Geometry: see drawing. Coordinates: mm, zero at the bounding-box minimum. Coordinates: 2 decimals unless noted, no trailing zeros. Write each loop counter-clockwise with the first axis right and the second up, starting at its lowest first coordinate (ties: lowest second). Pieces come first, ordered by that corner, then holes. Notation, with made-up numbers: M -33.75,-9 L -21.75,-9 A36 cw -21.75,26 Z; hole C 85,-28.75 d1. An arc over 180 degrees is marked long. One line per item, written item: value. Start each with the question number.
Item 1: Mould query, pull axis X, two halves, no side actions, for the marked faces 1, 2, 3 and 4. Classes: released by +X, released by -X, zero draft, split by the parting line, or undercut.
Item 2: Cut plane C-C, the plane y = 3.5. Output: boundary loops of the cut face in (x, z), then the cut area to 3 significant figures.
Item 3: Pin query (flat end, axial travel): P1, Ø6, axis at x = 12.5, y = 15.5, coming from the -Z side. Return the tip coordinate at first contact, or that it passes through.
Item 4: Cut plane A-A, the plane x = 12.5. Output: boundary loops of the cut face in (y, z).
Item 5: Cut plane D-D, the plane y = 15.25. Output: boundary loops of the cut face in (x, z).
Item 6: Ray query, L1, parallel to Y at x = 12.5, z = 24.5; L2, parallel to Y at x = 20.5, z = 10.5; L3, parallel to Y at x = 21, z = 16.75. Return the intervals inside material, ascending. Write a range as from..to.
Item 7: Cut plane B-B, the plane z = 15. Output: boundary loops of the cut face in (x, y).
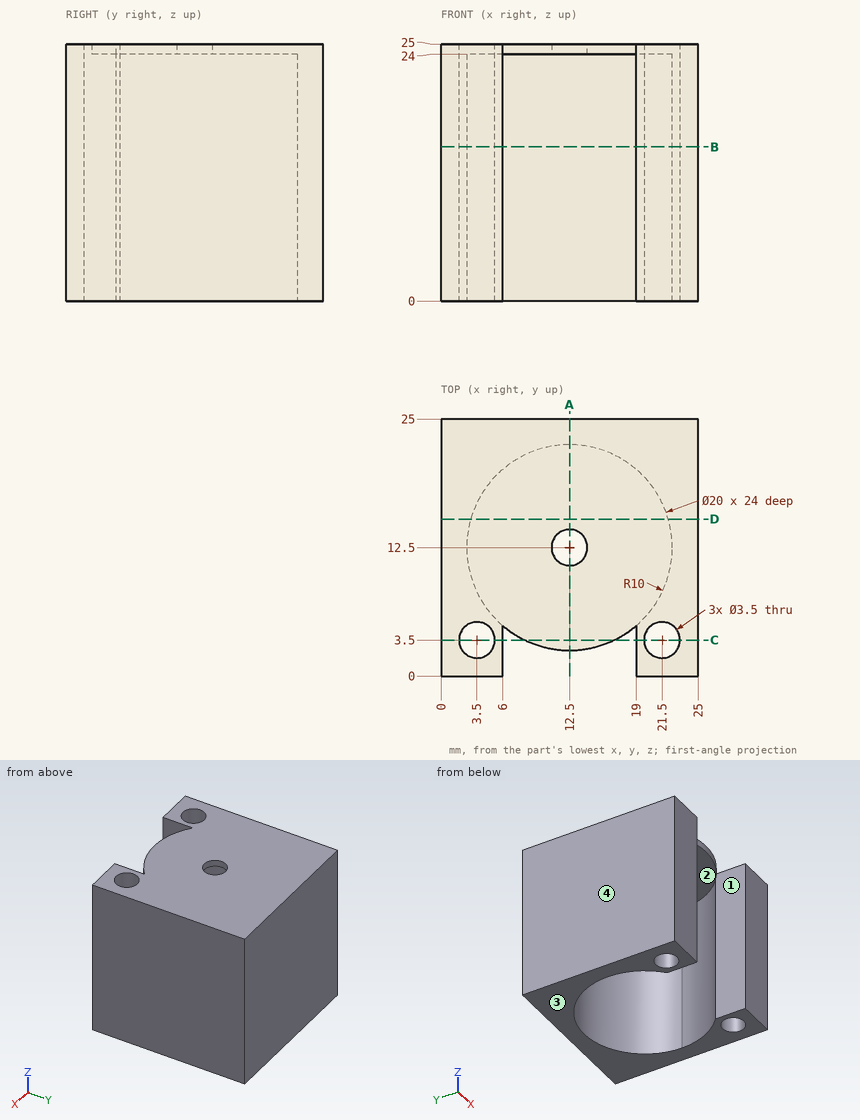
From the geometry:
1. face 1: undercut
1. face 2: undercut
1. face 3: zero draft
1. face 4: released by -X
2. outline: M 0,0 L 1.75,0 L 1.75,25 L 0,25 Z; M 5.25,0 L 6,0 L 6,25 L 5.25,25 Z; M 8.14,24 L 16.86,24 L 16.86,25 L 8.14,25 Z; M 19,0 L 19.75,0 L 19.75,25 L 19,25 Z; M 23.25,0 L 25,0 L 25,25 L 23.25,25 Z
2. area: 134 mm²
3. P1: stops at z = 24
4. outline: M 2.5,24 L 10.75,24 L 10.75,25 L 2.5,25 Z; M 14.25,24 L 22.5,24 L 22.5,0 L 25,0 L 25,25 L 14.25,25 Z
5. outline: M 0,0 L 2.89,0 L 2.89,24 L 22.11,24 L 22.11,0 L 25,0 L 25,25 L 0,25 Z
6. L1: y = 2.5..10.75, 14.25..25
6. L2: y = 0..2.06, 4.94..6.5, 18.5..25
6. L3: y = 0..1.82, 5.18..7.23, 17.77..25
7. outline: M 0,0 L 6,0 L 6,4.9 A10 cw long 19,4.9 L 19,0 L 25,0 L 25,25 L 0,25 Z; hole C 3.5,3.5 d3.5; hole C 21.5,3.5 d3.5
